Part model, mm, in its own coordinate system. A direction names the side the tool comes from. Give positions to 0.01 mm unless a question says otherwise; leave off trailing zeros. Loops run counter-clockwise (first coordinate to the right, second up) from the corner with the lowest first, then second, coordinate; pieces in that order, holes last. Notation, with made-up numbers: M 58.25,19.5 L 75.25,19.5 A26 cw 75.25,53.5 Z; hole C -36.5,-28 d5. An arc over 180 degrees is marked long. Answer in a Markdown table with one row per item.
from build123d import *

# Parameters (mm, degrees)
F0_W        = 150
F0_H        = 100
F1_DEPTH    = 95
F2_W        = 70
F2_H        = 45
F2_W_2      = 67
F2_W_3      = 46
F2_H_2      = 35
F2_W_4      = 65
F2_W_5      = 22
F3_DEPTH    = 90
F4_T1_DEPTH = 355.2081528017


# Not quite as in the source:
# - a fillet or chamfer that OpenCascade refuses, or shapes differently, is made with other operations: its cross-section is extruded or revolved along the edge and cut away or added


with BuildPart() as f1:
    # F0 (on Top) → F1 (new body)
    with BuildSketch(Plane.XY):
        with Locations((22.7672072938, 3.643443808)):
            Rectangle(F0_W, F0_H)
    extrude(amount=F1_DEPTH)

    # F2 (on face) → F3 (cut)
    with BuildSketch(Plane.XY.offset(95)):
        with Locations((-11, 25.1181102521)):
            Rectangle(F2_W, F2_H)
        with Locations((60.1440875874, 25.1181102521)):
            Rectangle(F2_W_2, F2_H)
        with Locations((-23, -22.0472425799)):
            Rectangle(F2_W_3, F2_H_2)
        with Locations((35.4433003601, -22.0472425799)):
            Rectangle(F2_W_4, F2_H_2)
        with Locations((82.6440875874, -22.0472425799)):
            Rectangle(F2_W_5, F2_H_2)
    extrude(amount=-F3_DEPTH, mode=Mode.SUBTRACT)

    # F4: fillet of radius 41.0416305603 on 2 edges, made by hand

    # F4_s2 → F4_t1 (cut)
    with BuildSketch(Plane.YZ.offset(-154.8368691071)):
        with BuildLine():
            ThreePointArc((-5.3149256317, 95), (-34.3357409119, 82.9791847198), (-46.356556192, 53.9583694397))
            Line((-46.356556192, 53.9583694397), (-46.356556192, 95))
            Line((-46.356556192, 95), (-5.3149256317, 95))
        make_face()
        with BuildLine():
            ThreePointArc((53.643443808, 53.9583694397), (41.6226285278, 82.9791847198), (12.6018132476, 95))
            Line((12.6018132476, 95), (53.643443808, 95))
            Line((53.643443808, 95), (53.643443808, 53.9583694397))
        make_face()
    extrude(amount=F4_T1_DEPTH, mode=Mode.SUBTRACT)


solid = f1.part
(1) Pin check, flat tips, straight feed: pin 1 Ø6.5 at (x, y) = (85, -17.5) entering from +Z; pin 2 Ø1.5 at (x, z) = (-36, 59.5) entering from -Y; pin 3 Ø6 at (x, z) = (30, 67.5) entering from -Y. Stop position of each tip, or through.
Recorded:
| item | result |
|---|---|
| pin 1 | stops at z = 5 |
| pin 2 | stops at y = -46.08 |
| pin 3 | stops at y = -44.98 |
(2) Which spindle directions (+Z, -Z, +X, -X, +Y, -Y) get a long thin tool onto all of the face, cutting with end or side? Do faces 1 (the face through (26.644, 25, 51)), 2 (the face through (22.417, -42.447, 71.44)). Say none if no direction does.
Recorded:
| item | result |
|---|---|
| face 1 | +Z |
| face 2 | +Z, +X, -X, -Y |
(3) Saw through at D-D (z = 69.5). Write the cut outline in (x, y), plus the area to 3 significant figures.
Recorded:
| item | result |
|---|---|
| outline | M -52.23,-43.3 L 97.77,-43.3 L 97.77,50.59 L -52.23,50.59 Z; hole M -46,-39.55 L 0,-39.55 L 0,-4.55 L -46,-4.55 Z; hole M -46,2.62 L 24,2.62 L 24,47.62 L -46,47.62 Z; hole M 2.94,-39.55 L 67.94,-39.55 L 67.94,-4.55 L 2.94,-4.55 Z; hole M 26.64,2.62 L 93.64,2.62 L 93.64,47.62 L 26.64,47.62 Z; hole M 71.64,-39.55 L 93.64,-39.55 L 93.64,-4.55 L 71.64,-4.55 Z |
| area | 3,260 mm^2 |
(4) Drill centre lines: line 1 along X through (y, z) = (17, 69.5); line 2 along Y through (x, z) = (50.5, 38); line 3 along X through (y, z) = (-7, 65.5). Where is each one in solid material? Low to high.
Recorded:
| item | result |
|---|---|
| line 1 | x = -52.23 to -46, 24 to 26.64, 93.64 to 97.77 |
| line 2 | y = -46.36 to -39.55, -4.55 to 2.62, 47.62 to 53.64 |
| line 3 | x = -52.23 to -46, 0 to 2.94, 67.94 to 71.64, 93.64 to 97.77 |
(5) Saw through at C-C (y = -12). Write the cut outline in (x, z), plus the area to 3 significant figures.
Recorded:
| item | result |
|---|---|
| outline | M -52.23,0 L 97.77,0 L 97.77,94.45 L 93.64,94.45 L 93.64,5 L 71.64,5 L 71.64,94.45 L 67.94,94.45 L 67.94,5 L 2.94,5 L 2.94,94.45 L 0,94.45 L 0,5 L -46,5 L -46,94.45 L -52.23,94.45 Z |
| area | 2,270 mm^2 |
(6) Pull direction Y, two halves, no side cores. Call faces 3 (the face through (97.767, 3, 47)), 4 (the face through (22.417, 52.284, 64.435)), 5 (the face through (-46, 25, 51)), 6 (the face through (22, -46.357, 27)): +Y half, -Y half, draft (parallel to the pull), parting line (faces both ways), or undercut.
Recorded:
| item | result |
|---|---|
| face 3 | draft |
| face 4 | +Y half |
| face 5 | undercut |
| face 6 | -Y half |
(7) Saw through at B-B (x = 60). Write the cut outline in (y, z).
Recorded:
| item | result |
|---|---|
| outline | M -46.36,0 L 53.64,0 L 53.64,53.96 A41.04 ccw 47.62,75.37 L 47.62,5 L 2.62,5 L 2.62,95 L -4.55,95 L -4.55,5 L -39.55,5 L -39.55,76.6 A41.04 ccw -46.36,53.96 Z |
(8) Saw through at A-A (z = 18). Write the cut outline in (x, y), plus the area to 3 significant figures.
Recorded:
| item | result |
|---|---|
| outline | M -52.23,-46.36 L 97.77,-46.36 L 97.77,53.64 L -52.23,53.64 Z; hole M -46,-39.55 L 0,-39.55 L 0,-4.55 L -46,-4.55 Z; hole M -46,2.62 L 24,2.62 L 24,47.62 L -46,47.62 Z; hole M 2.94,-39.55 L 67.94,-39.55 L 67.94,-4.55 L 2.94,-4.55 Z; hole M 26.64,2.62 L 93.64,2.62 L 93.64,47.62 L 26.64,47.62 Z; hole M 71.64,-39.55 L 93.64,-39.55 L 93.64,-4.55 L 71.64,-4.55 Z |
| area | 4,180 mm^2 |
